```python
from build123d import *

# Parameters (mm, degrees)
SKETCH1_W           = 11.8
SKETCH1_H           = 80
BOSS_EXTRUDE1_DEPTH = 1.5
SKETCH2_W           = 7.5
SKETCH2_H           = 80
SKETCH2_W_2         = 2.6
BOSS_EXTRUDE2_DEPTH = 6
SKETCH3_W           = 3.738034865
SKETCH3_H           = 43
SKETCH3_W_2         = 2.6
SKETCH3_H_2         = 24
CUT_EXTRUDE1_DEPTH  = 6


with BuildPart() as part:
    # Sketch1 → Boss-Extrude1 (new body)
    with BuildSketch(Plane(origin=(0, 0, 0), x_dir=(1, 0, 0), z_dir=(0, 1, 0))):
        with Locations((2.138034865, -38.013787639)):
            Rectangle(SKETCH1_W, SKETCH1_H)
    extrude(amount=BOSS_EXTRUDE1_DEPTH)

    # Sketch2 → Boss-Extrude2 (add)
    with BuildSketch(Plane(origin=(0, 1.5, 0), x_dir=(1, 0, 0), z_dir=(0, 1, 0))):
        with Locations((-0.011965135, -38.013787639)):
            Rectangle(SKETCH2_W, SKETCH2_H)
        with Locations((6.738034865, -38.013787639)):
            Rectangle(SKETCH2_W_2, SKETCH2_H)
    extrude(amount=BOSS_EXTRUDE2_DEPTH)

    # Sketch3 → Cut-Extrude1 (cut)
    with BuildSketch(Plane(origin=(0, 7.5, 0), x_dir=(1, 0, 0), z_dir=(0, 1, 0))):
        with Locations((1.869017433, -23.513787639)):
            Rectangle(SKETCH3_W, SKETCH3_H)
        with Locations((6.738034865, -14.013787639)):
            Rectangle(SKETCH3_W_2, SKETCH3_H_2)
    extrude(amount=-CUT_EXTRUDE1_DEPTH, mode=Mode.SUBTRACT)


solid = part.part
```
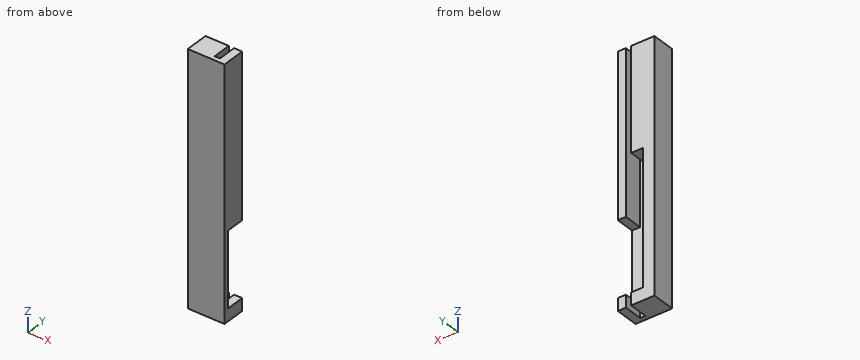
Geometry: final body of the model. Coordinates: model frame, mm. Coordinates: 2 decimals unless noted, no trailing zeros. Order: outer loops, then holes, each group sorted by start corner. A loop starts at its lowest first (then second) coordinate and runs counter-clockwise, first axis right, second up. Notation, with made-up numbers: (38, 53) -> (84, 53) arc R22 ccw to (84, 82) -> close; hole circle Ø1 at (88, -25.5). An arc over 180 degrees is marked (long way). Answer in a Markdown table with one row per item.
Item 1: Contact query for a flat-ended pin moving along its axis: P1, Ø3, axis at y = 5, z = 21.5, coming from the +X side. Output: stop coordinate, or through.
Return value:
| item | result |
|---|---|
| P1 | stops at x = 0 |
Item 2: Section C-C on z = 59.5. Output: boundary loops of the cut face in (x, y).
Return value:
| item | result |
|---|---|
| outline | (-3.76, 0) -> (8.04, 0) -> (8.04, 7.5) -> (5.44, 7.5) -> (5.44, 1.5) -> (3.74, 1.5) -> (3.74, 7.5) -> (-3.76, 7.5) -> close |
Item 3: Section D-D on z = 8. Output: boundary loops of the cut face in (x, y), plus the area to 3 significant figures.
Return value:
| item | result |
|---|---|
| outline | (-3.76, 0) -> (8.04, 0) -> (8.04, 1.5) -> (0, 1.5) -> (0, 7.5) -> (-3.76, 7.5) -> close |
| area | 40.3 mm² |
Item 4: Section A-A on y = 5.5. Output: boundary loops of the cut face in (x, z), plus the area to 3 significant figures.
Return value:
| item | result |
|---|---|
| outline | (-3.76, -1.99) -> (3.74, -1.99) -> (3.74, 2.01) -> (0, 2.01) -> (0, 45.01) -> (3.74, 45.01) -> (3.74, 78.01) -> (-3.76, 78.01) -> close; (5.44, -1.99) -> (8.04, -1.99) -> (8.04, 2.01) -> (5.44, 2.01) -> close; (5.44, 26.01) -> (8.04, 26.01) -> (8.04, 78.01) -> (5.44, 78.01) -> close |
| area | 585 mm² |
Item 5: Section B-B on x = 1. Output: boundary loops of the cut face in (y, z).
Return value:
| item | result |
|---|---|
| outline | (0, -1.99) -> (7.5, -1.99) -> (7.5, 2.01) -> (1.5, 2.01) -> (1.5, 45.01) -> (7.5, 45.01) -> (7.5, 78.01) -> (0, 78.01) -> close |
Item 6: Ray query, L1, parallel to X at y = 2.5, z = 62; L2, parallel to X at y = 4.5, z = 35; L3, parallel to Z at x = 1.75, y = 5.25. Return the intervals inside material, ascending.
Return value:
| item | result |
|---|---|
| L1 | x = -3.76 to 3.74, 5.44 to 8.04 |
| L2 | x = -3.76 to 0, 5.44 to 8.04 |
| L3 | z = -1.99 to 2.01, 45.01 to 78.01 |
